Design review of the part built by this model. Coordinates are the model's own, in mm. Face numbers are marked on the shaded views. A direction names the side the tool comes from. Give positions to 0.01 mm unless a question says otherwise; leave off trailing zeros. Loops run counter-clockwise (first coordinate to the right, second up) from the corner with the lowest first, then second, coordinate; pieces in that order, holes last. Notation, with made-up numbers: (-9.5, 35.25) -> (-5.5, 35.25) arc R12 cw to (-5.5, 46.25) -> close; hole circle Ø6 at (9, -25.5). An arc over 180 degrees is marked (long way). Use CSV: the item, a comma, the result in double quotes. Start each with the question number.
Item 1: We need section D-D (y = -8). State the section outline as (x, z) points.
Item 2: We need section A-A (x = 0). State the section outline as (y, z) points, plus the area to 3 significant figures.
Item 3: Wall thickness on line 1 along Y through (x, z) = (-4.5, 2.25); line 2 along Y through (x, z) = (3.5, -0.25); line 3 along X through (y, z) = (3.5, -3): over which ranges is each line inside the solid? List them lowest first. Write a range as from..to.
Item 4: For the marked faces 1, 2 and 3, list the 3-axis set-ups (+Z, -Z, +X, -X, +Y, -Y) from which the entire face can be reached by the end or side of a thin tool; tool diameter is ignored.
Item 5: We need section C-C (y = 5.25). State the section outline as (x, z) points.
Item 6: We need section B-B (z = 0). State the section outline as (x, y) points.
Item 7: Clearance check with flat-ended pins moving along their axes: pin 1 (1.5 mm diameter, centred on y = -3, z = -0.5, fed in from +X); pin 2 (2 mm diameter, centred on y = -5, z = 3, fed in from +X); pin 3 (4 mm diameter, centred on y = -4.5, z = 3, fed in from -X). State where each tip first meets the part, or that it passes through.
from build123d import *

# Parameters (mm, degrees)
SKETCH_1_W          = 10
SKETCH_1_H          = 10
EXTRUDE_1_DEPTH     = 11
SKETCH_2_R          = 4
EXTRUDE_2_DEPTH     = 18
SKETCH_3_W          = 2
SKETCH_3_H          = 10
CUT_EXTRUDE_1_DEPTH = 46
CUT_EXTRUDE_2_DEPTH = 46


with BuildPart() as part:
    # 草图1 → 凸台-拉伸1 (new body)
    with BuildSketch(Plane(origin=(0, 0, 0), x_dir=(1, 0, 0), z_dir=(0, 1, 0))):
        Rectangle(SKETCH_1_W, SKETCH_1_H)
    extrude(amount=EXTRUDE_1_DEPTH)

    # 草图2 → 凸台-拉伸2 (add)
    with BuildSketch(Plane.XZ):
        Circle(SKETCH_2_R)
    extrude(amount=EXTRUDE_2_DEPTH)

    # 草图3 → 切除-拉伸1 (cut)
    with BuildSketch(Plane.XY.offset(5)):
        with Locations((-4, 6)):
            Rectangle(SKETCH_3_W, SKETCH_3_H)
        with Locations((4, 6)):
            Rectangle(SKETCH_3_W, SKETCH_3_H)
    extrude(amount=-CUT_EXTRUDE_1_DEPTH, mode=Mode.SUBTRACT)

    # 草图4 → 切除-拉伸2 (cut)
    with BuildSketch(Plane(origin=(3, 0, 0), x_dir=(0, 0, -1), z_dir=(1, 0, 0))):
        with BuildLine():
            Line((-5, 6), (-5, 15.436246411))
            Line((-5, 15.436246411), (5, 15.436246411))
            Line((5, 15.436246411), (5, 6))
            ThreePointArc((5, 6), (0, 11), (-5, 6))
        make_face()
    extrude(amount=-CUT_EXTRUDE_2_DEPTH, mode=Mode.SUBTRACT)


solid = part.part
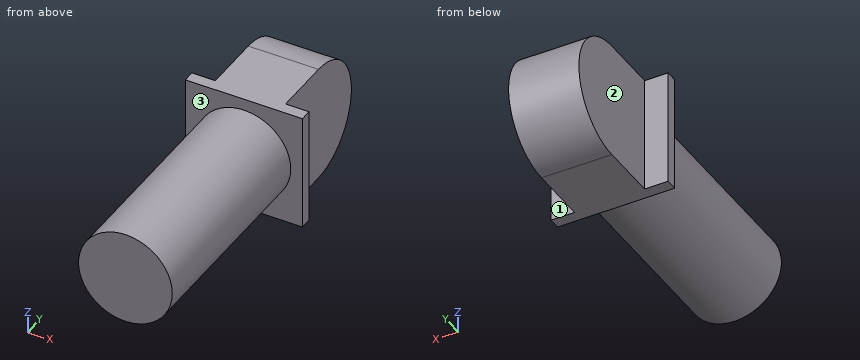
Results found:
1,outline,"circle Ø8 at (0, 0)"
2,outline,"(-18, -4) -> (0, -4) -> (0, -5) -> (6, -5) arc R5 ccw to (6, 5) -> (0, 5) -> (0, 4) -> (-18, 4) -> close"
2,area,"243 mm²"
3,line 1,"0..1"
3,line 2,"-18..1"
3,line 3,"-3..3"
4,face 1,"+Z, -Z, +X, +Y"
4,face 2,"+Z, -Z, -X, +Y"
4,face 3,"-Y"
5,outline,"(-3, -5) -> (3, -5) -> (3, 5) -> (-3, 5) -> close"
6,outline,"(-5, 0) -> (-4, 0) -> (-4, -18) -> (4, -18) -> (4, 0) -> (5, 0) -> (5, 1) -> (3, 1) -> (3, 11) -> (-3, 11) -> (-3, 1) -> (-5, 1) -> close"
7,pin 1,"x = 4"
7,pin 2,"x = 3.46"
7,pin 3,"x = -3.87"
